The model under review builds one solid part; all positions refer to its coordinate system, in mm. A direction names the side the tool comes from. Give positions to 0.01 mm unless a question says otherwise; leave off trailing zeros. Loops run counter-clockwise (first coordinate to the right, second up) from the corner with the lowest first, then second, coordinate; pieces in that order, holes last. Notation, with made-up numbers: (36.25, 75) -> (63.25, 75) arc R22 cw to (63.25, 83) -> close; hole circle Ø9 at (80, 87.5). An arc over 180 degrees is marked (long way). Write each question's results on one line, items separated by ' | '. Start each with the question number.
Q1. Insertion check: pin 1 Ø1.6 at (x, z) = (-38.5, 2) entering from -Y; pin 2 Ø2.5 at (y, z) = (-35, 3.5) entering from +X; pin 3 Ø2.5 at (x, z) = (31.5, 1.5) entering from +Y; pin 4 Ø12 at (x, y) = (-30.5, -10.5) entering from -Z. Each pin has a flat end and moves straight along its axis. Give the tip position at first contact, or say it passes through.
Q2. We need section C-C (x = 34.5). Write out the cut boundary in (y, z).
Q3. We need section A-A (z = 1.7). Write out the cut boundary in (x, y), plus the area to 3 significant figures.
Q4. Wall thickness on L1, parallel to X at y = -4, z = 3.6; L2, parallel to Y at x = 37, z = 1.4; L3, parallel to Y at x = 29.5, z = 1.3: over which ranges is each line inside the solid? List them lowest first. Write a range as [from, to].
Q5. We need section B-B (y = 5.5). Write out the cut boundary in (x, z), plus the area to 3 significant figures.
Q6. Machinability: for faces 1 (the face through (-12.7, -35, 3)), 2 (the face through (-12.7, 35, 3)), 3 (the face through (38, 16.7, 3)), which of the approach directions +Z, -Z, +X, -X, +Y, -Y give a long, thin tool a straight path to every point of the face, cutting with its end or side? Answer none if there is none.
Q7. Mouldability with a two-part tool opening along Y and no side actions: class faces 4 (the face through (-40.958, 25, 3)), 5 (the face through (-27, 32.575, 3)), 6 (the face through (-35.496, 0, 3)), 7 (the face through (-38, -16.7, 3)) as released by +Y, released by -Y, zero draft, split by the parting line, or undercut.
from build123d import *

# Parameters (mm, degrees)
SKETCH1_W           = 81.915
SKETCH1_H           = 65.151
BOSS_EXTRUDE1_DEPTH = 5.461
SKETCH2_W           = 5.461
SKETCH2_H           = 33.401
CUT_EXTRUDE1_DEPTH  = 6.461
SKETCH5_W           = 25.4
SKETCH5_H           = 5.461
BOSS_EXTRUDE2_DEPTH = 5.461


with BuildPart() as part:
    # Sketch1 → Boss-Extrude1 (new body)
    with BuildSketch(Plane.XY):
        Rectangle(SKETCH1_W, SKETCH1_H)
    extrude(amount=BOSS_EXTRUDE1_DEPTH)

    # Sketch2 → Cut-Extrude1 (cut, through all)
    with BuildSketch(Plane.XY.offset(5.461)):
        with Locations((-38.227, 0)):
            Rectangle(SKETCH2_W, SKETCH2_H)
        with Locations((38.227, 0)):
            Rectangle(SKETCH2_W, SKETCH2_H)
    extrude(amount=-CUT_EXTRUDE1_DEPTH, mode=Mode.SUBTRACT)

    # Sketch5 → Boss-Extrude2 (add)
    with BuildSketch(Plane(origin=(0, 0, 0), x_dir=(-1, 0, 0), z_dir=(0, 0, -1))):
        with Locations((0, 35.306)):
            Rectangle(SKETCH5_W, SKETCH5_H)
        with Locations((0, -35.306)):
            Rectangle(SKETCH5_W, SKETCH5_H)
    extrude(amount=-BOSS_EXTRUDE2_DEPTH)


solid = part.part
Output:
1) pin 1: y = -32.58 | pin 2: x = 12.7 | pin 3: y = 32.58 | pin 4: z = 0
2) outline: (-32.58, 0) -> (32.58, 0) -> (32.58, 5.46) -> (-32.58, 5.46) -> close
3) outline: (-40.96, -32.58) -> (-12.7, -32.58) -> (-12.7, -38.04) -> (12.7, -38.04) -> (12.7, -32.58) -> (40.96, -32.58) -> (40.96, -16.7) -> (35.5, -16.7) -> (35.5, 16.7) -> (40.96, 16.7) -> (40.96, 32.58) -> (12.7, 32.58) -> (12.7, 38.04) -> (-12.7, 38.04) -> (-12.7, 32.58) -> (-40.96, 32.58) -> (-40.96, 16.7) -> (-35.5, 16.7) -> (-35.5, -16.7) -> (-40.96, -16.7) -> close | area: 5,250 mm2
4) L1: [-35.5, 35.5] | L2: [-32.58, -16.7], [16.7, 32.58] | L3: [-32.58, 32.58]
5) outline: (-35.5, 0) -> (35.5, 0) -> (35.5, 5.46) -> (-35.5, 5.46) -> close | area: 388 mm2
6) face 1: +Z, -Z, -X, -Y | face 2: +Z, -Z, -X, +Y | face 3: +Z, -Z, +X
7) face 4: zero draft | face 5: released by +Y | face 6: undercut | face 7: undercut
